Source: CAD feature listing. Evaluate the final solid. Frame: model axes, mm. A direction names the side the tool comes from. Coordinates: 2 decimals unless noted, no trailing zeros. Write each loop counter-clockwise with the first axis right and the second up, starting at its lowest first coordinate (ties: lowest second). Pieces come first, ordered by that corner, then holes. Notation, with made-up numbers: (-35.5, -4.5) - (-24.5, -4.5) arc R25 cw to (-24.5, 16.5) - close; hole circle Ø5 at (-20.75, -4.5). An arc over 180 degrees is marked (long way). One line per question, with ' | ' between items.
from build123d import *

# Parameters (mm, degrees)
SKETCH1_R           = 1.932130595
SKETCH1_R_2         = 2.077751344
SKETCH1_R_3         = 2.074790544
SKETCH1_R_4         = 1.977245509
SKETCH1_W           = 37.994310796
SKETCH1_H           = 38.225983422
BOSS_EXTRUDE1_DEPTH = 5.08


with BuildPart() as part:
    # Sketch1 → Boss-Extrude1 (new body)
    with BuildSketch(Plane.XY):
        Polygon((-46.541317365, 64.792814371), (42.586826347, 64.792814371), (42.586826347, 45.932934132), (55.3889879, 45.932934132), (55.3889879, 33.156886228), (74.222754491, 33.156886228), (74.222754491, -55.971257485), (55.3889879, -55.971257485), (55.3889879, -68.652333238), (42.586826347, -68.652333238), (42.586826347, -87.607185629), (-46.541317365, -87.607185629), (-46.541317365, -68.652333238), (-59.317365269, -68.652333238), (-59.317365269, -55.971257485), (-78.177245509, -55.971257485), (-78.177245509, 33.156886228), (-59.317365269, 33.156886228), (-59.317365269, 45.932934132), (-46.541317365, 45.932934132), align=None)
        with Locations((-25.038400907, -11.407185629)):
            Circle(SKETCH1_R, mode=Mode.SUBTRACT)
        with Locations((-1.977245509, 11.769806082)):
            Circle(SKETCH1_R_2, mode=Mode.SUBTRACT)
        with Locations((21.083909889, -11.407185629)):
            Circle(SKETCH1_R_3, mode=Mode.SUBTRACT)
        with Locations((-1.977245509, -34.58417734)):
            Circle(SKETCH1_R_4, mode=Mode.SUBTRACT)
        with Locations((-1.977245509, -11.407185629)):
            Rectangle(SKETCH1_W, SKETCH1_H, mode=Mode.SUBTRACT)
    extrude(amount=BOSS_EXTRUDE1_DEPTH)


solid = part.part
Item 1: Pin query (flat end, axial travel): pin 1 Ø1.5 at (x, z) = (67, 1.5) entering from -Y; pin 2 Ø1.5 at (x, z) = (-51.5, 2) entering from +Y; pin 3 Ø1.5 at (x, z) = (67, 2) entering from +Y. Return the tip coordinate at first contact, or that it passes through.
Check sheet entries:
pin 1: y = -55.97 | pin 2: y = 45.93 | pin 3: y = 33.16
Item 2: Ray query, line 1 along X through (y, z) = (-11.5, 0.3); line 2 along Y through (x, z) = (12, 2.15); line 3 along X through (y, z) = (-6, 3.3). Return the intervals inside material, ascending. Write a range as [from, to].
Check sheet entries:
line 1: [-78.18, -26.97], [-23.11, -20.97], [17.02, 19.01], [23.16, 74.22] | line 2: [-87.61, -30.52], [7.71, 64.79] | line 3: [-78.18, -20.97], [17.02, 74.22]
Item 3: Cut plane B-B on z = 3.55. Return loops of the section in (x, y).
Check sheet entries:
outline: (-78.18, -55.97) - (-59.32, -55.97) - (-59.32, -68.65) - (-46.54, -68.65) - (-46.54, -87.61) - (42.59, -87.61) - (42.59, -68.65) - (55.39, -68.65) - (55.39, -55.97) - (74.22, -55.97) - (74.22, 33.16) - (55.39, 33.16) - (55.39, 45.93) - (42.59, 45.93) - (42.59, 64.79) - (-46.54, 64.79) - (-46.54, 45.93) - (-59.32, 45.93) - (-59.32, 33.16) - (-78.18, 33.16) - close; hole circle Ø3.86 at (-25.04, -11.41); hole (-20.97, -30.52) - (17.02, -30.52) - (17.02, 7.71) - (-20.97, 7.71) - close; hole circle Ø4.16 at (-1.98, 11.77); hole circle Ø3.95 at (-1.98, -34.58); hole circle Ø4.15 at (21.08, -11.41)
Item 4: Mould query, pull axis Y, two halves, no side actions, for faces 1 (the face through (-2.406, -36.514, 2.504)), 2 (the face through (55.389, -62, 3)), 3 (the face through (-69, 33.157, 3)). Classes: pulls with the +Y half, pulls with the -Y half, needs draft (parallel to the pull), parting line crosses it, or undercut.
Check sheet entries:
face 1: undercut | face 2: needs draft | face 3: pulls with the +Y half
Item 5: Cut plane C-C on y = -74. Return loops of the section in (x, z).
Check sheet entries:
outline: (-46.54, 0) - (42.59, 0) - (42.59, 5.08) - (-46.54, 5.08) - close
Item 6: Cut plane D-D on x = 50.5. Return loops of the section in (y, z).
Check sheet entries:
outline: (-68.65, 0) - (45.93, 0) - (45.93, 5.08) - (-68.65, 5.08) - close
Item 7: Cut plane A-A on x = 10.5. Return loops of the section in (y, z).
Check sheet entries:
outline: (-87.61, 0) - (-30.52, 0) - (-30.52, 5.08) - (-87.61, 5.08) - close; (7.71, 0) - (64.79, 0) - (64.79, 5.08) - (7.71, 5.08) - close
Item 8: Access query for faces 4 (the face through (-59.317, -62, 3)), 5 (the face through (-2, -30.52, 3)), 6 (the face through (-46.541, 55, 3)). Directions: +Z, -Z, +X, -X, +Y, -Y. A direction counts if a zero-diameter tool reaches every point of the face in a straight line with its end or side. Return the directions, or none.
Check sheet entries:
face 4: +Z, -Z, -X, -Y | face 5: +Z, -Z | face 6: +Z, -Z, -X, +Y
